Geometry check sheet. Reference: the model listing, model coordinates, mm. A direction names the side the tool comes from. Coordinates: 2 decimals unless noted, no trailing zeros. Write each loop counter-clockwise with the first axis right and the second up, starting at its lowest first coordinate (ties: lowest second). Pieces come first, ordered by that corner, then holes. Notation, with made-up numbers: M -34.75,-1 L 16.25,-1 A17 cw 16.25,9 Z; hole C -2,-31.75 d11. An arc over 180 degrees is marked long. Write each question's results on one line, items separated by ' | '.
```python
from build123d import *

# Parameters (mm, degrees)
SKETCH1_W           = 260
SKETCH1_H           = 260
SKETCH1_R           = 1.55
SKETCH1_R_2         = 1.5875
SKETCH1_R_3         = 1.6
SKETCH1_R_4         = 1.7
SKETCH1_R_5         = 2.415
SKETCH1_R_6         = 1.651
BOSS_EXTRUDE2_DEPTH = 6.35
SKETCH5_W           = 52.8
SKETCH5_H           = 52.8
CUT_EXTRUDE1_DEPTH  = 7.35
SKETCH6_R           = 3.175
CUT_EXTRUDE2_DEPTH  = 7.35
SKETCH7_R           = 1.5875
CUT_EXTRUDE3_DEPTH  = 7.35
SKETCH8_W           = 25.4
SKETCH8_H           = 6.35
SKETCH8_W_2         = 6.35
SKETCH8_H_2         = 25.4
CUT_EXTRUDE4_DEPTH  = 7.35


with BuildPart() as part:
    # Sketch1 → Boss-Extrude2 (new body)
    with BuildSketch(Plane.XY):
        Rectangle(SKETCH1_W, SKETCH1_H)
        with Locations((-26.035, 26.67)):
            Circle(SKETCH1_R, mode=Mode.SUBTRACT)
        with Locations((-26.035, -26.67)):
            Circle(SKETCH1_R, mode=Mode.SUBTRACT)
        with Locations((26.035, 26.67)):
            Circle(SKETCH1_R, mode=Mode.SUBTRACT)
        with Locations((26.035, -26.67)):
            Circle(SKETCH1_R, mode=Mode.SUBTRACT)
        with Locations((-124.036081104, 38.237690774)):
            Circle(SKETCH1_R_2, mode=Mode.SUBTRACT)
        with Locations((-120.861081104, -27.800206824)):
            Circle(SKETCH1_R_2, mode=Mode.SUBTRACT)
        with Locations((-75.776081104, 38.239793176)):
            Circle(SKETCH1_R_2, mode=Mode.SUBTRACT)
        with Locations((-37, 117)):
            Circle(SKETCH1_R_3, mode=Mode.SUBTRACT)
        with Locations((-37, 83)):
            Circle(SKETCH1_R_3, mode=Mode.SUBTRACT)
        with Locations((-3.5, 117)):
            Circle(SKETCH1_R_3, mode=Mode.SUBTRACT)
        with Locations((-3.5, 83)):
            Circle(SKETCH1_R_3, mode=Mode.SUBTRACT)
        with Locations((3.5, 117)):
            Circle(SKETCH1_R_3, mode=Mode.SUBTRACT)
        with Locations((37, 117)):
            Circle(SKETCH1_R_3, mode=Mode.SUBTRACT)
        with Locations((37, 83)):
            Circle(SKETCH1_R_3, mode=Mode.SUBTRACT)
        with Locations((3.5, 83)):
            Circle(SKETCH1_R_3, mode=Mode.SUBTRACT)
        with Locations((-13.25, -65.25)):
            Circle(SKETCH1_R_4, mode=Mode.SUBTRACT)
        with Locations((13.25, -65.25)):
            Circle(SKETCH1_R_4, mode=Mode.SUBTRACT)
        with Locations((13.25, -94.75)):
            Circle(SKETCH1_R_4, mode=Mode.SUBTRACT)
        with Locations((-13.25, -94.75)):
            Circle(SKETCH1_R_4, mode=Mode.SUBTRACT)
        with Locations((0, 55.575)):
            Circle(SKETCH1_R_5, mode=Mode.SUBTRACT)
        with Locations((-55.575, 0)):
            Circle(SKETCH1_R_5, mode=Mode.SUBTRACT)
        with Locations((0, -55.575)):
            Circle(SKETCH1_R_5, mode=Mode.SUBTRACT)
        with Locations((55.575, 0)):
            Circle(SKETCH1_R_5, mode=Mode.SUBTRACT)
        with Locations((-39.297459364, 39.297459364)):
            Circle(SKETCH1_R_5, mode=Mode.SUBTRACT)
        with Locations((39.297459364, 39.297459364)):
            Circle(SKETCH1_R_5, mode=Mode.SUBTRACT)
        with Locations((39.297459364, -39.297459364)):
            Circle(SKETCH1_R_5, mode=Mode.SUBTRACT)
        with Locations((-39.297459364, -39.297459364)):
            Circle(SKETCH1_R_5, mode=Mode.SUBTRACT)
        with Locations((-78.951081104, -27.800206824)):
            Circle(SKETCH1_R_2, mode=Mode.SUBTRACT)
        with Locations((6.35, -121.3)):
            Circle(SKETCH1_R_6, mode=Mode.SUBTRACT)
        with Locations((-6.35, -121.3)):
            Circle(SKETCH1_R_6, mode=Mode.SUBTRACT)
        with Locations((121.3, 126.35)):
            Circle(SKETCH1_R_6, mode=Mode.SUBTRACT)
        with Locations((121.3, 113.65)):
            Circle(SKETCH1_R_6, mode=Mode.SUBTRACT)
    extrude(amount=BOSS_EXTRUDE2_DEPTH)

    # Sketch5 → Cut-Extrude1 (cut, through all)
    with BuildSketch(Plane(origin=(0, 0, 0), x_dir=(-1, 0, 0), z_dir=(0, 0, -1))):
        with Locations((-104.6, 104.6)):
            Rectangle(SKETCH5_W, SKETCH5_H)
    extrude(amount=-CUT_EXTRUDE1_DEPTH, mode=Mode.SUBTRACT)

    # Sketch6 → Cut-Extrude2 (cut, through all)
    with BuildSketch(Plane(origin=(0, 0, 0), x_dir=(-1, 0, 0), z_dir=(0, 0, -1))):
        with Locations((63.77864005, 63.77864005)):
            Circle(SKETCH6_R)
        with Locations((-63.87464005, 63.77864005)):
            Circle(SKETCH6_R)
        with Locations((-63.87464005, -63.87464005)):
            Circle(SKETCH6_R)
        with Locations((63.77864005, -63.87464005)):
            Circle(SKETCH6_R)
    extrude(amount=-CUT_EXTRUDE2_DEPTH, mode=Mode.SUBTRACT)

    # Sketch7 → Cut-Extrude3 (cut, through all)
    with BuildSketch(Plane(origin=(0, 0, 0), x_dir=(-1, 0, 0), z_dir=(0, 0, -1))):
        with Locations((91.9, 118.189)):
            Circle(SKETCH7_R)
        with Locations((104.6, 118.189)):
            Circle(SKETCH7_R)
        with Locations((117.3, 118.189)):
            Circle(SKETCH7_R)
        with Locations((91.9, -45.133)):
            Circle(SKETCH7_R)
        with Locations((104.6, -45.133)):
            Circle(SKETCH7_R)
        with Locations((117.3, -45.133)):
            Circle(SKETCH7_R)
        with Locations((45.133, -117.3)):
            Circle(SKETCH7_R)
        with Locations((45.133, -104.6)):
            Circle(SKETCH7_R)
        with Locations((45.133, -91.9)):
            Circle(SKETCH7_R)
        with Locations((-118.189, -117.3)):
            Circle(SKETCH7_R)
        with Locations((-118.189, -104.6)):
            Circle(SKETCH7_R)
        with Locations((-118.189, -91.9)):
            Circle(SKETCH7_R)
    extrude(amount=-CUT_EXTRUDE3_DEPTH, mode=Mode.SUBTRACT)

    # Sketch8 → Cut-Extrude4 (cut, through all)
    with BuildSketch(Plane.XY.offset(6.35)):
        with Locations((-102.241050682, -62.663768992)):
            Rectangle(SKETCH8_W, SKETCH8_H)
        with Locations((-64.693745391, 92.61029866)):
            Rectangle(SKETCH8_W_2, SKETCH8_H_2)
        with Locations((101.629283102, 59.681030297)):
            Rectangle(SKETCH8_W_2, SKETCH8_H_2)
    extrude(amount=-CUT_EXTRUDE4_DEPTH, mode=Mode.SUBTRACT)


solid = part.part
```
Q1. Sectioned sample at A-A on y = 99. Record the cut outline in (x, z), and give its area (3 significant figures).
Geometry check:
outline: M -130,0 L -67.87,0 L -67.87,6.35 L -130,6.35 Z; M -61.52,0 L 78.2,0 L 78.2,6.35 L -61.52,6.35 Z | area: 1,280 mm2
Q2. Sectioned sample at C-C on z = 2. Give the number of separate pieces and of enclosed holes in the cut face, and give its area (3 significant figures).
Geometry check:
separate pieces: 1 | enclosed holes: 49 | area: 63,900 mm2
Q3. Sectioned sample at B-B on x = 111. Record the cut outline in (y, z).
Geometry check:
outline: M -130,0 L 78.2,0 L 78.2,6.35 L -130,6.35 Z
Q4. Scan lines: probe 1 along Y at (x, z) = (-45, 4.75); probe 2 along X at (y, z) = (-66.5, 5.5); probe 3 along Y at (x, z) = (37.5, 0.75). Record each from-to range of solid material in increasing order.
Geometry check:
probe 1: y = -130 to -118.88, -115.72 to -106.18, -103.02 to -93.48, -90.32 to 130 | probe 2: x = -130 to -65.56, -61.99 to -14.4, -12.1 to 12.1, 14.4 to 62.09, 65.66 to 130 | probe 3: y = -130 to -40.91, -37.68 to 37.68, 40.91 to 81.48, 84.52 to 115.48, 118.52 to 130
Q5. Depth check by flat-ended pin: P1, Ø3, axis at x = -55.575, y = 0, coming from the +Z side; P2, Ø7.5, axis at x = 39.3, y = 39.3, coming from the -Z side. Enter the tip coordinate at first touch or a pass-through.
Geometry check:
P1: passes through | P2: stops at z = 0
Q6. Access from +Z, -Z, +X, -X, +Y, -Y to the whole of each face (thin tool, end or side, straight path). Record for faces 1 (the flat face through (78.2, 104, 3)), 2 (the flat face through (-2, 2, 6.35)), 3 (the flat face through (-65, 105.31, 3)).
Geometry check:
face 1: +Z, -Z, +X, +Y | face 2: +Z, +X, -X, +Y, -Y | face 3: +Z, -Z
